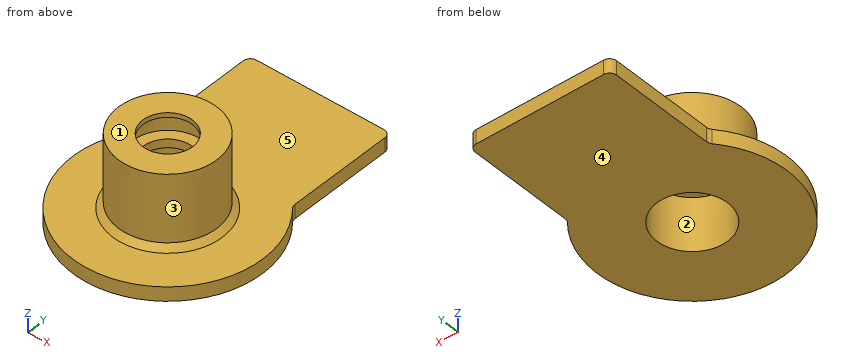
from build123d import *

# Parameters (mm, degrees)
BOSS_EXTRUDE1_DEPTH = 2
FILLET2_R           = 1
CHAMFER1_SIZE       = 0.8


with BuildPart() as part:
    # Sketch2 → Revolve1 (revolve)
    with BuildSketch(Plane(origin=(0, 0, 0), x_dir=(1, 0, 0), z_dir=(0, 1, 0))):
        Polygon((-3.5, -12.32), (-3.5, -11.68), (-4.925, -11.2), (-4.925, -8.7), (-3.45, -8.7), (-3.45, -7.5), (-5, -7.5), (-5, 0), (-13.4, 0), (-13.4, -2), (-6.925, -2), (-6.925, -12.32), align=None)
    revolve(axis=Axis((0, 0, 0), (0, 0, 1)))

    # Sketch3 → Boss-Extrude1 (add)
    with BuildSketch(Plane.XY.offset(2)):
        with BuildLine():
            Line((10, 8.919641248), (10, 25.121576202))
            Line((10, 25.121576202), (-10, 25.121576202))
            Line((-10, 25.121576202), (-10, 8.919641248))
            ThreePointArc((-10, 8.919641248), (0, 13.4), (10, 8.919641248))
        make_face()
    extrude(amount=-BOSS_EXTRUDE1_DEPTH)

    # Fillet2
    fillet2_edges = [part.edges().sort_by_distance(p)[0] for p in [
        (10, 25.121576202, 1),
        (-10, 25.121576202, 1),
        (-10, 8.919641248, 1),
        (10, 8.919641248, 1),
    ]]
    fillet(fillet2_edges, radius=FILLET2_R)

    # Chamfer1
    chamfer1_edges = [part.edges().sort_by_distance(p)[0] for p in [
        (6.925, 0, 2),
    ]]
    chamfer(chamfer1_edges, length=CHAMFER1_SIZE)


solid = part.part
Source: CAD feature listing. Evaluate the final solid. Frame: model axes, mm. Face numbers are marked on the shaded views. A direction names the side the tool comes from. Give positions to 0.01 mm unless a question says otherwise; leave off trailing zeros. Write each loop counter-clockwise with the first axis right and the second up, starting at its lowest first coordinate (ties: lowest second). Pieces come first, ordered by that corner, then holes. Notation, with made-up numbers: (-35.75, 82.5) - (16.25, 82.5) arc R22 cw to (16.25, 95.5) - close; hole circle Ø4 at (29, -39). An arc over 180 degrees is marked (long way). Write item = value, one per line. Start each with the question number.
Q1. Cut plane B-B, the plane x = 0. Return loops of the section in (y, z) (3 decimals), then the cut area to 3 significant figures.
Q2. Cut plane A-A, the plane y = 0. Return loops of the section in (x, z) (3 decimals).
Q3. Draft query along Y for the marked faces 1, 2 and 3. Return one class per face: +Y half, -Y half, draft (parallel to the pull), parting line (faces both ways), or undercut.
Q4. Reachability of the marked faces 4 and 5 from +Z, -Z, +X, -X, +Y, -Y: full face, straight path, thin tool, end or side. Return the list, or none.
Q5. Cut plane D-D, the plane y = 13. Return loops of the section in (x, z).
Q6. Cut plane C-C, the plane z = 6. Return loops of the section in (x, y) (3 decimals), then the cut area to 3 significant figures.
Q7. Material intervals for probe 1 along Y at (x, z) = (0, 9.85) (3 decimals); probe 2 along Y at (x, z) = (0, 12.1) (3 decimals), sorted ascending.
Q8. Pin query (flat end, axial travel): pin 1 Ø1.6 at (y, z) = (14, 1) entering from -X; pin 2 Ø3 at (y, z) = (-5.5, 7) entering from +X; pin 3 Ø4 at (x, y) = (-4, 19.5) entering from +Z. Return the tip coordinate at first contact, or that it passes through.
Computed values:
q1.outline = (-13.4, 0) - (-5, 0) - (-5, 7.5) - (-3.45, 7.5) - (-3.45, 8.7) - (-4.925, 8.7) - (-4.925, 11.2) - (-3.5, 11.68) - (-3.5, 12.32) - (-6.925, 12.32) - (-6.925, 2.8) - (-7.725, 2) - (-13.4, 2) - close; (3.45, 7.5) - (5, 7.5) - (5, 0) - (25.122, 0) - (25.122, 2) - (7.725, 2) - (6.925, 2.8) - (6.925, 12.32) - (3.5, 12.32) - (3.5, 11.68) - (4.925, 11.2) - (4.925, 8.7) - (3.45, 8.7) - close
q1.area = 104 mm²
q2.outline = (-13.4, 0) - (-5, 0) - (-5, 7.5) - (-3.45, 7.5) - (-3.45, 8.7) - (-4.925, 8.7) - (-4.925, 11.2) - (-3.5, 11.68) - (-3.5, 12.32) - (-6.925, 12.32) - (-6.925, 2.8) - (-7.725, 2) - (-13.4, 2) - close; (3.45, 7.5) - (5, 7.5) - (5, 0) - (13.4, 0) - (13.4, 2) - (7.725, 2) - (6.925, 2.8) - (6.925, 12.32) - (3.5, 12.32) - (3.5, 11.68) - (4.925, 11.2) - (4.925, 8.7) - (3.45, 8.7) - close
q3.face_1 = draft
q3.face_2 = undercut
q3.face_3 = parting line
q4.face_4 = -Z, +X, -X, +Y, -Y
q4.face_5 = +Z
q5.outline = (-10, 0) - (10, 0) - (10, 2) - (-10, 2) - close
q6.outline = circle Ø13.85 at (0, 0); hole circle Ø10 at (0, 0)
q6.area = 72.1 mm²
q7.probe_1 = -6.925 to -4.925, 4.925 to 6.925
q7.probe_2 = -6.925 to -3.5, 3.5 to 6.925
q8.pin_1 = -10
q8.pin_2 = 5.65
q8.pin_3 = 2
